Read the model definition and answer for the solid it produces. Units are mm, in the model's axes. Round coordinates to 2 decimals unless told otherwise and drop trailing zeros. Order: outer loops, then holes, each group sorted by start corner. A loop starts at its lowest first (then second) coordinate and runs counter-clockwise, first axis right, second up. Notation, with made-up numbers: (39.5, 80.5) - (46.5, 80.5) arc R17 ccw to (46.5, 104.5) - close; hole circle Ø9 at (-14.5, 33.5). An arc over 180 degrees is marked (long way). One line per question, with ' | ' between items. Start each with the question number.
1) Straight lines are drawn through the part: line 1 (X direction, y = -4, z = 170); line 2 (Y direction, x = 6.45, z = 75). For each, find the intervals that lie inside material, in ascending order. Write a range as from..to.
2) A flat-ended cylindrical pin translates along its axis: pin 1 (3.5 mm diameter, centred on x = 0, z = 7.5, fed in from -Y). Find the tip coordinate at first contact, or state that the pin passes through.
3) The part is cut by section B-B, the plane y = 0. Give the vertices of the cut face in (x, z), plus the area to 3 significant figures.
4) The part is cut by section C-C, the plane x = 0. Count the separate pieces of the cut face and the enclosed holes in it, plus the area to 3 significant figures.
5) The part is cut by section A-A, the plane z = 22.5. Give the vertices of the cut face in (x, y).
6) The part is cut by section D-D, the plane z = 56. Give the vertices of the cut face in (x, y), plus the area to 3 significant figures.
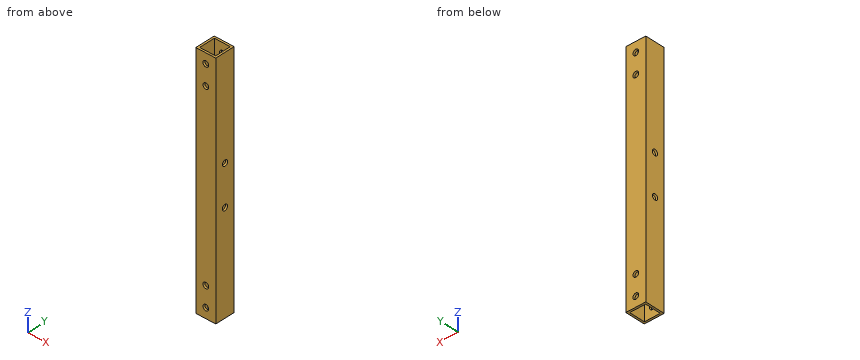
from build123d import *

# Parameters (mm, degrees)
SKETCH_1_W          = 15
SKETCH_1_H          = 15
SKETCH_1_W_2        = 12
SKETCH_1_H_2        = 12
EXTRUDE_1_DEPTH     = 180
SKETCH_3_R          = 2.15
CUT_EXTRUDE_2_DEPTH = 181.779561898
SKETCH_4_R          = 2.15
CUT_EXTRUDE_3_DEPTH = 181.779561898


with BuildPart() as part:
    # ｽｹｯﾁ1 → 押し出し-薄板1 (new body)
    with BuildSketch(Plane.XY):
        Rectangle(SKETCH_1_W, SKETCH_1_H)
        Rectangle(SKETCH_1_W_2, SKETCH_1_H_2, mode=Mode.SUBTRACT)
    extrude(amount=EXTRUDE_1_DEPTH)

    # ｽｹｯﾁ3 → ｶｯﾄ - 押し出し2 (cut, through all)
    with BuildSketch(Plane(origin=(7.5, 0, 0), x_dir=(0, 0, -1), z_dir=(1, 0, 0))):
        with Locations((-75, 0)):
            Circle(SKETCH_3_R)
        with Locations((-105, 0)):
            Circle(SKETCH_3_R)
    extrude(amount=-CUT_EXTRUDE_2_DEPTH, mode=Mode.SUBTRACT)

    # ｽｹｯﾁ4 → ｶｯﾄ - 押し出し3 (cut, through all)
    with BuildSketch(Plane(origin=(0, 7.5, 0), x_dir=(1, 0, 0), z_dir=(0, 1, 0))):
        with Locations(Location((0, -7.5, 0), (0, 0, 270))):
            Circle(SKETCH_4_R)
        with Locations(Location((0, -22.5, 0), (0, 0, 270))):
            Circle(SKETCH_4_R)
        with Locations(Location((0, -172.5, 0), (0, 0, 270))):
            Circle(SKETCH_4_R)
        with Locations(Location((0, -157.5, 0), (0, 0, 270))):
            Circle(SKETCH_4_R)
    extrude(amount=-CUT_EXTRUDE_3_DEPTH, mode=Mode.SUBTRACT)


solid = part.part
Values:
1) line 1: x = -7.5..-6, 6..7.5 | line 2: y = -7.5..-2.15, 2.15..7.5
2) pin 1: passes through
3) outline: (-7.5, 0) - (-6, 0) - (-6, 72.85) - (-7.5, 72.85) - close; (-7.5, 77.15) - (-6, 77.15) - (-6, 102.85) - (-7.5, 102.85) - close; (-7.5, 107.15) - (-6, 107.15) - (-6, 180) - (-7.5, 180) - close; (6, 0) - (7.5, 0) - (7.5, 72.85) - (6, 72.85) - close; (6, 77.15) - (7.5, 77.15) - (7.5, 102.85) - (6, 102.85) - close; (6, 107.15) - (7.5, 107.15) - (7.5, 180) - (6, 180) - close | area: 514 mm^2
4) separate pieces: 10 | enclosed holes: 0 | area: 488 mm^2
5) outline: (-7.5, -7.5) - (-2.15, -7.5) - (-2.15, -6) - (-6, -6) - (-6, 6) - (-2.15, 6) - (-2.15, 7.5) - (-7.5, 7.5) - close; (2.15, -7.5) - (7.5, -7.5) - (7.5, 7.5) - (2.15, 7.5) - (2.15, 6) - (6, 6) - (6, -6) - (2.15, -6) - close
6) outline: (-7.5, -7.5) - (7.5, -7.5) - (7.5, 7.5) - (-7.5, 7.5) - close; hole (-6, -6) - (6, -6) - (6, 6) - (-6, 6) - close | area: 81.0 mm^2
